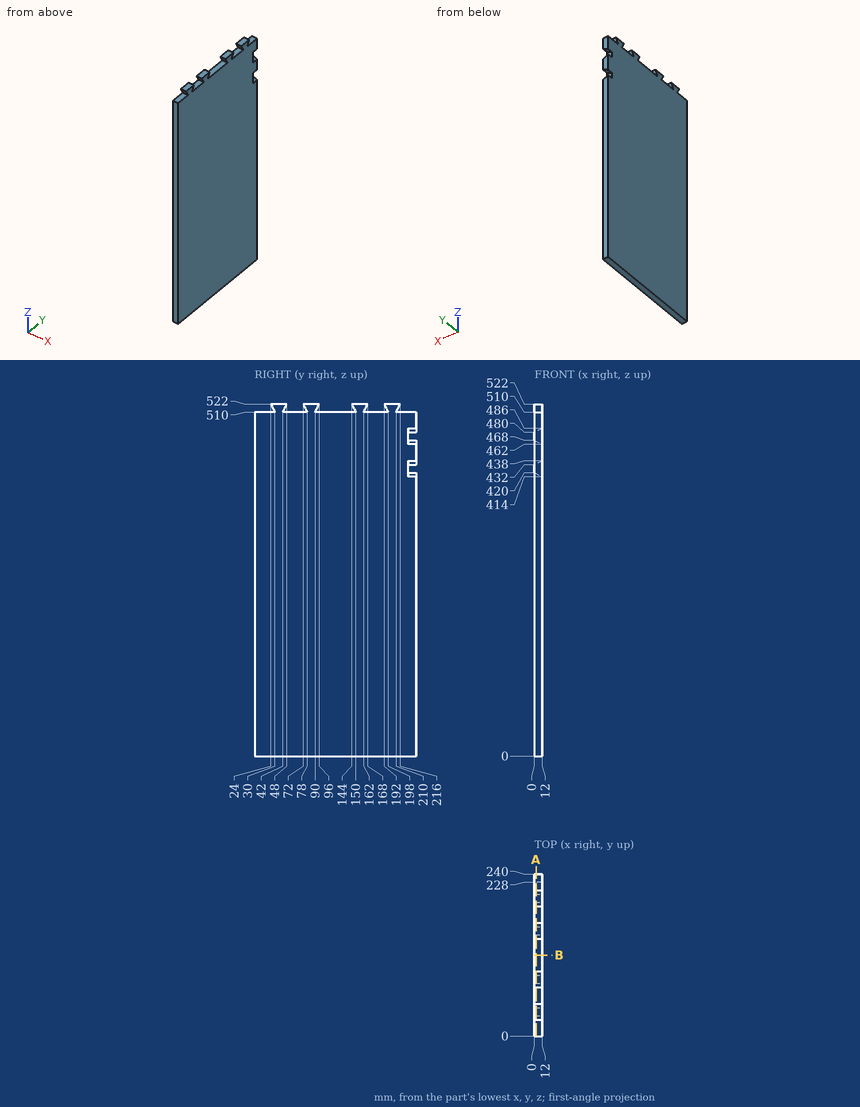
Input: dimensioned drawing with shaded views. Units: mm. Origin: part minimum x, y, z. Round coordinates to 2 decimals unless told otherwise and drop trailing zeros. Loops run counter-clockwise (first coordinate to the right, second up) from the corner with the lowest first, then second, coordinate; pieces in that order, holes last. Notation, with made-up numbers: (57, 48.5) -> (78, 48.5) arc R20 cw to (78, 78.5) -> close; hole circle Ø2 at (-17.5, 18.5). An arc over 180 degrees is marked (long way). Answer as a JSON object with one key per item and string values. Group by question number.
1) Section query B-B on y = 120. Output: boundary loops of the cut face in (x, z), plus the area to 3 significant figures.
2) Pin query (flat end, axial travel): pin 1 (1.5 mm diameter, centred on x = 4, y = 103, fed in from -Z); pin 2 (3 mm diameter, centred on x = 9.5, y = 62.5, fed in from +Z); pin 3 (6 mm diameter, centred on x = 8, z = 429.5, fed in from +Y). Return the tip coordinate at first contact, or that it passes through.
3) Ray query, L1, parallel to Y at x = 6.5, z = 482.5; L2, parallel to Z at x = 7.25, y = 221; L3, parallel to Z at x = 5.75, y = 215.5. Return the intervals inside material, ascending.
4) Section query A-A on x = 2.5. Output: boundary loops of the cut face in (y, z).
Reply:
{
 "1": {"outline": "(0, 0) -> (12, 0) -> (12, 510) -> (0, 510) -> close", "area": "6,120 mm2"},
 "2": {"pin 1": "stops at z = 0", "pin 2": "stops at z = 510", "pin 3": "stops at y = 228"},
 "3": {"L1": "y = 0 to 228", "L2": "z = 0 to 510", "L3": "z = 0 to 510, 521 to 522"},
 "4": {"outline": "(0, 0) -> (240, 0) -> (240, 418.75) -> (228, 418.75) -> (228, 433.25) -> (240, 433.25) -> (240, 466.75) -> (228, 466.75) -> (228, 481.25) -> (240, 481.25) -> (240, 510) -> (210, 510) -> (216, 522) -> (192, 522) -> (198, 510) -> (162, 510) -> (168, 522) -> (144, 522) -> (150, 510) -> (90, 510) -> (96, 522) -> (72, 522) -> (78, 510) -> (42, 510) -> (48, 522) -> (24, 522) -> (30, 510) -> (0, 510) -> close"}
}
